```python
from build123d import *

# Parameters (mm, degrees)
SKETCH_1_R          = 11
EXTRUDE_1_DEPTH     = 2
EXTRUDE_START       = -2
SKETCH_2_R          = 1.6
EXTRUDE_2_DEPTH     = 2
CUT_EXTRUDE_1_REACH = 25.545
SKETCH_3_R          = 1.6
SKETCH_4_R          = 8.75
SKETCH_4_R_2        = 7.15
EXTRUDE_3_DEPTH     = 3


with BuildPart() as part:
    # 草图1 → 凸台-拉伸1 (new body)
    with BuildSketch(Plane(origin=(0, 0, 0), x_dir=(1, 0, 0), z_dir=(0, 1, 0))):
        with Locations(Location((0, 0, 0), (0, 0, 270))):
            Circle(SKETCH_1_R)
    extrude(amount=EXTRUDE_1_DEPTH)

    # 草图2 → 凸台-拉伸2 (add)
    # profile 1 of 3: a face of its own
    with BuildSketch(Plane(origin=(0, 2, 0), x_dir=(1, 0, 0), z_dir=(0, 1, 0)).offset(EXTRUDE_START)):
        with BuildLine():
            ThreePointArc((0.053619854, -10.999869313), (5.5, -9.526279442), (9.499356337, -5.546370812))
            ThreePointArc((9.499356337, -5.546370812), (8.961509488, -7.8135778), (9.778378275, -9.995831713))
            ThreePointArc((9.778378275, -9.995831713), (8.75, -15.155444566), (3.767455058, -13.466239851))
            ThreePointArc((3.767455058, -13.466239851), (2.286002125, -11.667683773), (0.053619854, -10.999869313))
        make_face()
        with Locations(Location((7, -12.124355653, 0), (0, 0, 270))):
            Circle(SKETCH_2_R, mode=Mode.SUBTRACT)
    # profile 2 of 3: a face of its own
    with BuildSketch(Plane(origin=(0, 2, 0), x_dir=(1, 0, 0), z_dir=(0, 1, 0)).offset(EXTRUDE_START)):
        with BuildLine():
            ThreePointArc((9.499356337, 5.546370812), (5.5, 9.526279442), (0.053619854, 10.999869313))
            ThreePointArc((0.053619854, 10.999869313), (2.286002125, 11.667683773), (3.767455058, 13.466239851))
            ThreePointArc((3.767455058, 13.466239851), (8.75, 15.155444566), (9.778378275, 9.995831713))
            ThreePointArc((9.778378275, 9.995831713), (8.961509488, 7.8135778), (9.499356337, 5.546370812))
        make_face()
        with Locations(Location((7, 12.124355653, 0), (0, 0, 270))):
            Circle(SKETCH_2_R, mode=Mode.SUBTRACT)
    # profile 3 of 3: a face of its own
    with BuildSketch(Plane(origin=(0, 2, 0), x_dir=(1, 0, 0), z_dir=(0, 1, 0)).offset(EXTRUDE_START)):
        with BuildLine():
            ThreePointArc((-9.55297619, -5.453498501), (-11.247511613, -3.854105973), (-13.545833333, -3.470408137))
            ThreePointArc((-13.545833333, -3.470408137), (-17.5, 0), (-13.545833333, 3.470408137))
            ThreePointArc((-13.545833333, 3.470408137), (-11.247511613, 3.854105973), (-9.55297619, 5.453498501))
            ThreePointArc((-9.55297619, 5.453498501), (-11, 0), (-9.55297619, -5.453498501))
        make_face()
        with Locations(Location((-14, 0, 0), (0, 0, 270))):
            Circle(SKETCH_2_R, mode=Mode.SUBTRACT)
    extrude(amount=EXTRUDE_2_DEPTH)

    # 草图3 → 切除-拉伸1 (cut, up to next)
    with BuildSketch(Plane(origin=(0, 2, 0), x_dir=(1, 0, 0), z_dir=(0, 1, 0)), mode=Mode.PRIVATE) as cut_extrude_1_sk1:
        with Locations(Location((0, 0, 0), (0, 0, 270))):
            Circle(SKETCH_3_R)
    cut_extrude_1_tool1 = extrude(cut_extrude_1_sk1.sketch, amount=-CUT_EXTRUDE_1_REACH, mode=Mode.PRIVATE) & part.part
    add(cut_extrude_1_tool1.solids().sort_by_distance((0, 2, 0))[0], mode=Mode.SUBTRACT)

    # 草图4 → 凸台-拉伸3 (add)
    with BuildSketch(Plane(origin=(0, 2, 0), x_dir=(1, 0, 0), z_dir=(0, 1, 0))):
        with Locations(Location((0, 0, 0), (0, 0, 270))):
            Circle(SKETCH_4_R)
        with Locations(Location((0, 0, 0), (0, 0, 270))):
            Circle(SKETCH_4_R_2, mode=Mode.SUBTRACT)
    extrude(amount=EXTRUDE_3_DEPTH)


solid = part.part
```
Model file for the job. Use its own axes, mm. A direction names the side the tool comes from. Give positions to 0.01 mm unless a question says otherwise; leave off trailing zeros. Loops run counter-clockwise (first coordinate to the right, second up) from the corner with the lowest first, then second, coordinate; pieces in that order, holes last. Notation, with made-up numbers: (16, 36.5) - (45, 36.5) arc R23 cw to (45, 46.5) - close; hole circle Ø7 at (71, -18.75). An arc over 180 degrees is marked (long way). One line per item, written item: value. Start each with the question number.
1. Pull direction X, two halves, no side cores. Call faces 3 (the cylindrical face through (5.58, 0.99, -11.39)), 4 (the cylindrical face through (-12.414, 0.986, -0.208)), 5 (the cylindrical face through (-5.324, 3.479, -6.944)), 6 (the flat face through (3, 0, 0)): pulls with the +X half, pulls with the -X half, needs draft (parallel to the pull), parting line crosses it, or undercut.
2. Slice it at B-B (z = 0). List the corners of the cut face in (x, y), plus the area to 3 significant figures.
3. Which spindle directions (+Z, -Z, +X, -X, +Y, -Y) get a long thin tool onto all of the face, cutting with end or side? Do faces 1 (the cylindrical face through (5.438, 0.986, 11.778)), 2 (the flat face through (8, 2, -4)). Say none if no direction does.
4. Slice it at D-D (z = -6.5). List the corners of the cut face in (x, y), plus the area to 3 significant figures.
5. Slice it at A-A (x = -14). List the corners of the cut face in (y, z), plus the area to 3 significant figures.
6. Pin check, flat tips, straight feed: pin 1 (1.9 mm diameter, centred on x = 7, z = 12.12, fed in from +Y); pin 2 (1 mm diameter, centred on y = 2, z = -4.5, fed in from +X); pin 3 (5 mm diameter, centred on x = 3, z = -2, fed in from +Y). Stop position of each tip, or through.
7. Slice it at C-C (x = 6.5). List the corners of the cut face in (y, z).
8. Probe L1, parallel to X at y = 3.1, z = 0; L2, parallel to Y at x = 9, z = 11.5; L3, parallel to Z at x = -1.25, y = 3.35. List the from-to ranges inside material, lowest first. Write a range as from..to.
Solution:
1. face 3: undercut
1. face 4: undercut
1. face 5: parting line crosses it
1. face 6: needs draft
2. outline: (-17.5, 0) - (-15.6, 0) - (-15.6, 2) - (-17.5, 2) - close; (-12.4, 0) - (-1.6, 0) - (-1.6, 2) - (-7.15, 2) - (-7.15, 5) - (-8.75, 5) - (-8.75, 2) - (-12.4, 2) - close; (1.6, 0) - (11, 0) - (11, 2) - (8.75, 2) - (8.75, 5) - (7.15, 5) - (7.15, 2) - (1.6, 2) - close
2. area: 53.8 mm^2
3. face 1: +Y, -Y
3. face 2: +Y
4. outline: (-8.87, 0) - (9.1, 0) - (9.1, 2) - (5.86, 2) - (5.86, 5) - (2.98, 5) - (2.98, 2) - (-2.98, 2) - (-2.98, 5) - (-5.86, 5) - (-5.86, 2) - (-8.87, 2) - close
4. area: 53.2 mm^2
5. outline: (0, -3.5) - (2, -3.5) - (2, -1.6) - (0, -1.6) - close; (0, 1.6) - (2, 1.6) - (2, 3.5) - (0, 3.5) - close
5. area: 7.60 mm^2
6. pin 1: passes through
6. pin 2: stops at x = 10.25
6. pin 3: stops at y = 2
7. outline: (0, -15.59) - (2, -15.59) - (2, -13.64) - (0, -13.64) - close; (0, -10.6) - (2, -10.6) - (2, -5.86) - (5, -5.86) - (5, -2.98) - (2, -2.98) - (2, 2.98) - (5, 2.98) - (5, 5.86) - (2, 5.86) - (2, 10.6) - (0, 10.6) - close; (0, 13.64) - (2, 13.64) - (2, 15.59) - (0, 15.59) - close
8. L1: x = -8.75..-7.15, 7.15..8.75
8. L2: y = 0..2
8. L3: z = -8.66..-7.04, 7.04..8.66
